CAD build for the part. Positions are in the model's coordinates, mm. A direction names the side the tool comes from. Round coordinates to 2 decimals unless told otherwise and drop trailing zeros. Order: outer loops, then holes, each group sorted by start corner. A loop starts at its lowest first (then second) coordinate and runs counter-clockwise, first axis right, second up. Notation, with made-up numbers: (34, 54) - (41, 54) arc R21 cw to (41, 73) - close; hole circle Ø4 at (-26.5, 12.5). An arc over 180 degrees is marked (long way). Write item = value, one per line.
from build123d import *

# Parameters (mm, degrees)
F0_W     = 12
F0_H     = 22
F1_DEPTH = 22
F3_DEPTH = 4
F4_R     = 3
F5_DEPTH = 2
F7_DEPTH = 2
F8_R     = 1


with BuildPart() as f1:
    # F0 (on Top) → F1 (new body)
    with BuildSketch(Plane.XY):
        with Locations((-18.318631, 0.362903)):
            Rectangle(F0_W, F0_H)
    extrude(amount=F1_DEPTH)

    # F2 (on face) → F3 (join)
    with BuildSketch(Plane.XY.offset(22)):
        with BuildLine():
            ThreePointArc((-24.318631, 5.236689), (-18.318631, -0.763311), (-12.318631, 5.236689))
            ThreePointArc((-12.318631, 5.236689), (-18.318631, 11.236689), (-24.318631, 5.236689))
        make_face()
    extrude(amount=F3_DEPTH)

    # F4 (on face) → F5 (join)
    with BuildSketch(Plane.XY.offset(26)):
        with Locations((-18.318631, 5.236689)):
            Circle(F4_R)
    extrude(amount=F5_DEPTH)

    # F6 (on face) → F7 (join)
    with BuildSketch(Plane.XY.offset(28)):
        with BuildLine():
            Line((-18.318631, 20.221412), (-16.273675, 20.221412))
            ThreePointArc((-16.273675, 20.221412), (-18.318631, 22.266367), (-20.363586, 20.221412))
            Line((-20.363586, 20.221412), (-18.318631, 20.221412))
        make_face()
        with BuildLine():
            Line((-18.318631, 20.221412), (-20.363586, 20.221412))
            Line((-20.363586, 20.221412), (-21.253275, 5.859475))
            ThreePointArc((-21.253275, 5.859475), (-20.206969, 7.567822), (-18.318631, 8.236689))
            Line((-18.318631, 8.236689), (-18.318631, 20.221412))
        make_face()
        with BuildLine():
            Line((-15.383986, 5.859475), (-16.273675, 20.221412))
            Line((-16.273675, 20.221412), (-18.318631, 20.221412))
            Line((-18.318631, 20.221412), (-18.318631, 8.236689))
            ThreePointArc((-18.318631, 8.236689), (-16.430293, 7.567822), (-15.383986, 5.859475))
        make_face()
        with BuildLine():
            Line((-15.383986, 4.613903), (-15.383986, 5.859475))
            ThreePointArc((-15.383986, 5.859475), (-16.430293, 7.567822), (-18.318631, 8.236689))
            ThreePointArc((-18.318631, 8.236689), (-20.206969, 7.567822), (-21.253275, 5.859475))
            Line((-21.253275, 5.859475), (-21.253275, 4.613903))
            ThreePointArc((-21.253275, 4.613903), (-18.318631, 2.236689), (-15.383986, 4.613903))
        make_face()
        with BuildLine():
            Line((-16.273675, -9.748033), (-15.383986, 4.613903))
            ThreePointArc((-15.383986, 4.613903), (-18.318631, 2.236689), (-21.253275, 4.613903))
            Line((-21.253275, 4.613903), (-20.363586, -9.748033))
            Line((-20.363586, -9.748033), (-18.318631, -9.748033))
            Line((-18.318631, -9.748033), (-16.273675, -9.748033))
        make_face()
        with BuildLine():
            ThreePointArc((-20.363586, -9.748033), (-18.318631, -11.792988), (-16.273675, -9.748033))
            Line((-16.273675, -9.748033), (-18.318631, -9.748033))
            Line((-18.318631, -9.748033), (-20.363586, -9.748033))
        make_face()
    extrude(amount=F7_DEPTH)

    # F8
    f8_edges = [f1.edges().sort_by_distance(p)[0] for p in [
        (-12.318631, 11.362903, 11),
        (-24.318631, 11.362903, 11),
        (-12.318631, -10.637097, 11),
        (-24.318631, -10.637097, 11),
    ]]
    fillet(f8_edges, radius=F8_R)


solid = f1.part
(1) Probe line 1 along Z through (x, y) = (-17, 8.5); line 2 along Z through (x, y) = (-23.5, -8.5); line 3 along Z through (x, y) = (-19.5, 14). List the from-to ranges inside material, lowest first.
Solved:
line_1 = 0 to 26, 28 to 30
line_2 = 0 to 22
line_3 = 28 to 30
(2) Drop flat-ended pins along their axis: pin 1 (4 mm diameter, centred on x = -18, z = 18, fed in from -Y); pin 2 (1 mm diameter, centred on x = -14, y = 0.5, fed in from +Z); pin 3 (5 mm diameter, centred on x = -19, z = 8, fed in from +Y); pin 4 (4.5 mm diameter, centred on x = -18.5, y = 10.5, fed in from -Z). Give the stop position or say it passes through.
Solved:
pin_1 = -10.64
pin_2 = 26
pin_3 = 11.36
pin_4 = 0
(3) Band-saw the part on B-B on x = -17. List the corners of the cut face in (y, z).
Solved:
outline = (-11.31, 28) - (2.54, 28) - (2.54, 26) - (-0.62, 26) - (-0.62, 22) - (-10.64, 22) - (-10.64, 0) - (11.36, 0) - (11.36, 22) - (11.09, 22) - (11.09, 26) - (7.93, 26) - (7.93, 28) - (21.78, 28) - (21.78, 30) - (-11.31, 30) - close
(4) Band-saw the part on A-A on y = 0. List the corners of the cut face in (x, z).
Solved:
outline = (-24.32, 0) - (-12.32, 0) - (-12.32, 22) - (-15.39, 22) - (-15.39, 26) - (-21.25, 26) - (-21.25, 22) - (-24.32, 22) - close; (-20.97, 28) - (-15.67, 28) - (-15.67, 30) - (-20.97, 30) - close
(5) Tool access for faces 1 (the flat face through (-15.835, -2.668, 28.986)), 2 (the flat face through (-21.253, 5, 29)), 3 (the flat face through (-20.802, 13.141, 28.986)), 4 (the flat face through (-15.823, 12.94, 28.986)), 5 (the cylindrical face through (-12.776, 2.939, 23.972)): list every direction of +Z, -Z, +X, -X, +Y, -Y with a clear straight run to the whole face (end or side of a thin tool).
Solved:
face_1 = +Z, +X, -Y
face_2 = +Z, -X, +Y, -Y
face_3 = +Z, -X, +Y
face_4 = +Z, +X, +Y
face_5 = none
(6) Band-saw the part on C-C on z = 10. List the corners of the cut face in (x, y), plus the area to 3 significant figures.
Solved:
outline = (-24.32, -9.64) arc R1 ccw to (-23.32, -10.64) - (-13.32, -10.64) arc R1 ccw to (-12.32, -9.64) - (-12.32, 10.36) arc R1 ccw to (-13.32, 11.36) - (-23.32, 11.36) arc R1 ccw to (-24.32, 10.36) - close
area = 263 mm²
(7) Pull direction Z, two halves, no side cores. Call faces 6 (the cylindrical face through (-15.547, 4.088, 26.986)), 7 (the flat face through (-20.815, -2.467, 28.986)), 8 (the flat face through (-18, 5, 30)): released by +Z, released by -Z, zero draft, split by the parting line, or undercut.
Solved:
face_6 = undercut
face_7 = zero draft
face_8 = released by +Z
(8) Band-saw the part on D-D on y = -4.5. List the corners of the cut face in (x, z).
Solved:
outline = (-24.32, 0) - (-12.32, 0) - (-12.32, 22) - (-24.32, 22) - close; (-20.69, 28) - (-15.95, 28) - (-15.95, 30) - (-20.69, 30) - close
